Source: CAD feature listing. Evaluate the final solid. Frame: model axes, mm. A direction names the side the tool comes from. Give positions to 0.01 mm unless a question says otherwise; leave off trailing zeros. Write each loop counter-clockwise with the first axis right and the second up, starting at its lowest first coordinate (ties: lowest second). Pieces come first, ordered by that corner, then holes.
```python
from build123d import *

# Parameters (mm, degrees)
F1_W     = 127
F1_H     = 76.2
F1_R     = 12.7
F2_DEPTH = 25.4
F3_W     = 21.082
F3_H     = 76.2
F4_DEPTH = 15.24
F6_DEPTH = 76.201
F7_R     = 8.0634907525
F8_DEPTH = 25.4


with BuildPart() as f2:
    # F1 (on face) → F2 (new body)
    with BuildSketch(Plane.XY):
        Rectangle(F1_W, F1_H)
        Circle(F1_R, mode=Mode.SUBTRACT)
    extrude(amount=F2_DEPTH)

    # F3 (on face) → F4 (cut)
    with BuildSketch(Plane.XY.offset(25.4)):
        with Locations((-41.783, 0)):
            Rectangle(F3_W, F3_H)
        with BuildLine():
            Line((5.0697553696, 38.1), (-5.0902446304, 38.1))
            Line((-5.0902446304, 38.1), (-5.0902446304, 11.6352657728))
            ThreePointArc((-5.0902446304, 11.6352657728), (-0.0111778089, 12.699995081), (5.0697553696, 11.6442080234))
            Line((5.0697553696, 11.6442080234), (5.0697553696, 38.1))
        make_face()
        with BuildLine():
            Line((-5.0902446304, -11.6352657728), (-5.0902446304, -38.1))
            Line((-5.0902446304, -38.1), (5.0697553696, -38.1))
            Line((5.0697553696, -38.1), (5.0697553696, -11.6442080234))
            ThreePointArc((5.0697553696, -11.6442080234), (-0.0111778089, -12.699995081), (-5.0902446304, -11.6352657728))
        make_face()
    extrude(amount=-F4_DEPTH, mode=Mode.SUBTRACT)

    # F5 (on face) → F6 (cut, through all)
    with BuildSketch(Plane.XZ.offset(38.1)):
        Polygon((31.7397553696, 25.4), (19.0397553696, 25.4), (11.7074069509, 12.7), (39.0721037883, 12.7), align=None)
    extrude(amount=-F6_DEPTH, mode=Mode.SUBTRACT)

    # F7 (on face) → F8 (join)
    with BuildSketch(Plane.YZ.offset(63.5)):
        with Locations((0, 12.7)):
            Circle(F7_R)
    extrude(amount=F8_DEPTH)


solid = f2.part
```
1. Section query A-A (x = 0). Return loops of the section in (y, z).
2. Section query C-C (y = -2). Return loops of the section in (x, z).
3. Line query: probe 1 along X at (y, z) = (-27.5, 12.75); probe 2 along X at (y, z) = (-11, 14.5); probe 3 along X at (y, z) = (0, 11.75). Output: solid intervals per line, ascending.
4. Pin query (flat end, axial travel): P1, Ø7.5, axis at y = 26, z = 19.5, coming from the +X side; P2, Ø17, axis at x = -42, y = -1.5, coming from the +Z side; P3, Ø5, axis at x = 66.5, z = 22.5, coming from the +Y side. Return the tip coordinate at first contact, or that it passes through.
5. Pull-direction query (X, two-part tool) for faces 4 (the flat face through (-31.242, -1, 18)), 5 (the flat face through (47, 1, 25.4)), 6 (the flat face through (-63.5, -1, 13)); classes: pulls with the +X half, pulls with the -X half, needs draft (parallel to the pull), parting line crosses it, or undercut.
6. Access query for faces 1 (the flat face through (88.9, 0, 13)), 2 (the flat face through (15.425, -0.533, 19.139)), 3 (the flat face through (-52.324, -1, 18)). Directions: +Z, -Z, +X, -X, +Y, -Y. A direction counts if a zero-diameter tool reaches every point of the face in a straight line with its end or side. Return the directions, or none.
7. Section query B-B (z = 2.5). Return loops of the section in (x, y).
8. Section query D-D (y = 17.5). Return loops of the section in (x, z), plus the area to 3 significant figures.
The answers:
1. outline: (-38.1, 0) - (-12.7, 0) - (-12.7, 10.16) - (-38.1, 10.16) - close; (12.7, 0) - (38.1, 0) - (38.1, 10.16) - (12.7, 10.16) - close
2. outline: (-63.5, 0) - (-12.54, 0) - (-12.54, 25.4) - (-31.24, 25.4) - (-31.24, 10.16) - (-52.32, 10.16) - (-52.32, 25.4) - (-63.5, 25.4) - close; (12.54, 0) - (63.5, 0) - (63.5, 4.89) - (88.9, 4.89) - (88.9, 20.51) - (63.5, 20.51) - (63.5, 25.4) - (31.74, 25.4) - (39.07, 12.7) - (12.54, 12.7) - close; (12.54, 14.14) - (19.04, 25.4) - (12.54, 25.4) - close
3. probe 1: x = -63.5 to -52.32, -31.24 to -5.09, 5.07 to 11.74, 39.04 to 63.5
3. probe 2: x = -63.5 to -52.32, -31.24 to -6.35, 6.35 to 12.75, 38.03 to 63.5
3. probe 3: x = -63.5 to -52.32, -31.24 to -12.7, 12.7 to 88.9
4. P1: stops at x = 63.5
4. P2: stops at z = 10.16
4. P3: stops at y = 3.42
5. face 4: undercut
5. face 5: needs draft
5. face 6: pulls with the -X half
6. face 1: +Z, -Z, +X, +Y, -Y
6. face 2: +Y, -Y
6. face 3: +Z, +Y, -Y
7. outline: (-63.5, -38.1) - (63.5, -38.1) - (63.5, 38.1) - (-63.5, 38.1) - close; hole circle Ø25.4 at (0, 0)
8. outline: (-63.5, 0) - (63.5, 0) - (63.5, 25.4) - (31.74, 25.4) - (39.07, 12.7) - (11.71, 12.7) - (19.04, 25.4) - (5.07, 25.4) - (5.07, 10.16) - (-5.09, 10.16) - (-5.09, 25.4) - (-31.24, 25.4) - (-31.24, 10.16) - (-52.32, 10.16) - (-52.32, 25.4) - (-63.5, 25.4) - close
8. area: 2,500 mm2
